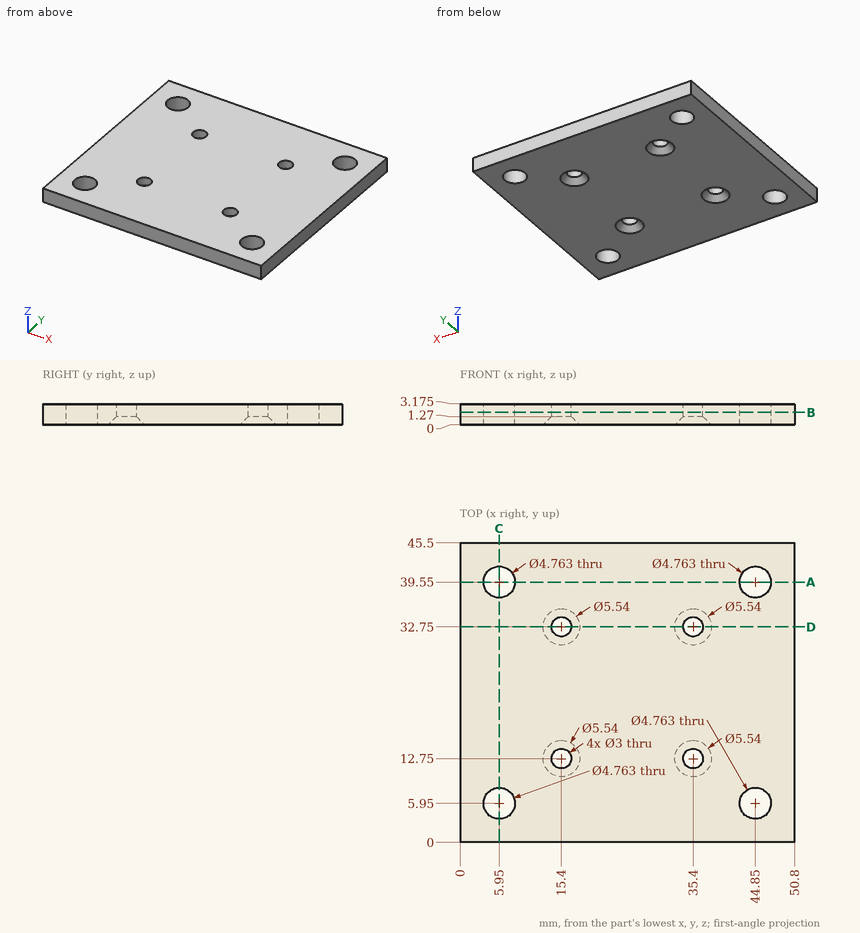
Here's the drawing with two shaded views (mm, measured from the low corner). I have some questions. Coordinates: 2 decimals unless noted, no trailing zeros. Write each loop counter-clockwise with the first axis right and the second up, starting at its lowest first coordinate (ties: lowest second). Pieces come first, ordered by that corner, then holes.
Item 1: If I drill on line 1 (X direction, y = 5.95, z = 0.8); line 2 (X direction, y = 32.75, z = 2.4); line 3 (Y direction, x = 6, z = 0.95), over which ranges is the centre line in solid material (lowest first)?
Item 2: I want a section at C-C on x = 5.95. Write out the boundary of the cut face in (y, z) (1 decimal).
Item 3: I want a section at B-B on z = 1.9. Count the separate pieces of the cut face and the enclosed holes in it, and give its area (3 significant figures).
Item 4: Will these pins go through, and if not, where does the flat tip stop? pin 1 (3.5 mm diameter, centred on x = 35.4, y = 32.75, fed in from -Z); pin 2 (4 mm diameter, centred on x = 15.4, y = 12.75, fed in from -Z).
Item 5: I want a section at D-D on y = 32.75. Write out the boundary of the cut face in (x, z) (1 decimal).
Item 6: I want a section at A-A on y = 39.55. Write out the boundary of the cut face in (x, z) (1 decimal).
Findings below:
1. line 1: x = 0 to 3.57, 8.33 to 42.47, 47.23 to 50.8
1. line 2: x = 0 to 13.9, 16.9 to 33.9, 36.9 to 50.8
1. line 3: y = 0 to 3.57, 8.33 to 37.17, 41.93 to 45.5
2. outline: (0, 0) - (3.6, 0) - (3.6, 3.2) - (0, 3.2) - close; (8.3, 0) - (37.2, 0) - (37.2, 3.2) - (8.3, 3.2) - close; (41.9, 0) - (45.5, 0) - (45.5, 3.2) - (41.9, 3.2) - close
3. separate pieces: 1
3. enclosed holes: 8
3. area: 2,210 mm2
4. pin 1: stops at z = 1.02
4. pin 2: stops at z = 0.77
5. outline: (0, 0) - (12.6, 0) - (13.9, 1.3) - (13.9, 3.2) - (0, 3.2) - close; (16.9, 1.3) - (18.2, 0) - (32.6, 0) - (33.9, 1.3) - (33.9, 3.2) - (16.9, 3.2) - close; (36.9, 1.3) - (38.2, 0) - (50.8, 0) - (50.8, 3.2) - (36.9, 3.2) - close
6. outline: (0, 0) - (3.6, 0) - (3.6, 3.2) - (0, 3.2) - close; (8.3, 0) - (42.5, 0) - (42.5, 3.2) - (8.3, 3.2) - close; (47.2, 0) - (50.8, 0) - (50.8, 3.2) - (47.2, 3.2) - close
